Source: CAD feature listing. Evaluate the final solid. Frame: model axes, mm. A direction names the side the tool comes from. Give positions to 0.01 mm unless a question says otherwise; leave off trailing zeros. Order: outer loops, then holes, each group sorted by start corner. A loop starts at its lowest first (then second) coordinate and runs counter-clockwise, first axis right, second up.
1) Section C-C, the plane x = 3.5. Return loops of the section in (y, z) (1 decimal).
2) Material intervals for line 1 (Z direction, x = 19, y = 5.25) (1 decimal); line 2 (Y direction, x = 2, z = 7); line 3 (Z direction, x = 3, y = -2.5), sorted ascending.
3) Access query for faces 1 (the face through (19, 0, -11.112)), 2 (the face through (11, 2.413, 0)), 3 (the face through (14.713, 10, 5)). Directions: +Z, -Z, +X, -X, +Y, -Y. A direction counts if a zero-diameter tool reaches every point of the face in a straight line with its end or side. Return the directions, or none.
4) Draft query along X for faces 4 (the face through (9.22, 2.89, -8.49)), 5 (the face through (11, -8.763, -1)), 6 (the face through (7.307, 0, -12)). Return one class per face: released by +X, released by -X, zero draft, split by the parting line, or undercut.
5) First-contact query: P1, Ø11.5, axis at x = 12, z = -11, coming from the +Y side; P2, Ø1.5, axis at y = 11, z = 7.5, coming from the -X side. Flat tips, straight axial feed; report the tip coordinate or a pass-through.
6) Section A-A, the plane y = -6.5. Return loops of the section in (x, z) (1 decimal), plus the area to 3 significant figures.
7) Section B-B, the plane x = 10.25. Give the number of separate pieces and of enclosed holes in the cut face, plus the area to 4 significant figures.
8) Section D-D, the plane z = -9. Return loops of the section in (x, y) (3 decimals).
```python
from build123d import *

# Parameters (mm, degrees)
SKETCH1_W                       = 22.225
SKETCH1_H                       = 17.526
BOSS_EXTRUDE1_DEPTH             = 22.225
SKETCH2_W                       = 7.874
SKETCH2_H                       = 17.526
BOSS_EXTRUDE2_DEPTH             = 2.54
SKETCH3_W                       = 22.225
SKETCH3_H                       = 6.35
CUT_EXTRUDE1_DEPTH              = 6.35
SKETCH5_W                       = 7.874
SKETCH5_H                       = 7.9375
BOSS_EXTRUDE3_DEPTH             = 5.08
F_1_4_20_START                  = -13.6525
F_1_4_20_TAPPED_HOLE1_OUTLINE_R = 2.5527
F_1_4_20_TAPPED_HOLE1_DEPTH     = 10.4775
CUT_EXTRUDE3_REACH              = 26.382
F_1_4_20_START_2                = 4.410249561
F_1_4_20_TAPPED_HOLE2_OUTLINE_R = 2.5527
F_1_4_20_TAPPED_HOLE2_DEPTH     = 8.960808925
SKETCH21_W                      = 0.508
SKETCH21_H                      = 3.96875
BOSS_EXTRUDE4_DEPTH             = 0.02
LPATTERN1_COUNT                 = 3
LPATTERN1_PITCH                 = 6.5
SKETCH22_W                      = 0.211811424
SKETCH22_H                      = 2.54
BOSS_EXTRUDE5_DEPTH             = 0.02
LPATTERN2_COUNT                 = 5
LPATTERN2_PITCH                 = 1.016
SKETCH23_W                      = 0.254
SKETCH23_H                      = 2.54
BOSS_EXTRUDE6_DEPTH             = 0.02
LPATTERN3_COUNT                 = 5
LPATTERN3_PITCH                 = 1


# Read off the part's stored shape, not the designer's step: 1/4-20 Tapped Hole1, 1/4-20 Tapped Hole2
with BuildPart() as part:
    # Sketch1 → Boss-Extrude1 (new body)
    with BuildSketch(Plane(origin=(0, 0, 0), x_dir=(0, 0, -1), z_dir=(1, 0, 0))):
        Rectangle(SKETCH1_W, SKETCH1_H)
    extrude(amount=BOSS_EXTRUDE1_DEPTH)

    # Sketch2 → Boss-Extrude2 (add)
    with BuildSketch(Plane(origin=(0, 0, -11.1125), x_dir=(-1, 0, 0), z_dir=(0, 0, -1))):
        with Locations((-11.243689687, 0)):
            Rectangle(SKETCH2_W, SKETCH2_H)
    extrude(amount=BOSS_EXTRUDE2_DEPTH)

    # Sketch3 → Cut-Extrude1 (cut)
    with BuildSketch(Plane(origin=(0, 8.763, 0), x_dir=(1, 0, 0), z_dir=(0, 1, 0))):
        with Locations((11.1125, 0)):
            Rectangle(SKETCH3_W, SKETCH3_H)
    extrude(amount=-CUT_EXTRUDE1_DEPTH, mode=Mode.SUBTRACT)

    # Sketch5 → Boss-Extrude3 (add)
    with BuildSketch(Plane(origin=(0, 8.763, 0), x_dir=(1, 0, 0), z_dir=(0, 1, 0))):
        with Locations((10.776161326, -7.14375)):
            Rectangle(SKETCH5_W, SKETCH5_H)
    extrude(amount=BOSS_EXTRUDE3_DEPTH)

    # 1/4-20 Tapped Hole1 outline → 1/4-20 Tapped Hole1 (cut)
    with BuildSketch(Plane.XY.offset(F_1_4_20_START)):
        with Locations((11.243689687, 4.445)):
            Circle(F_1_4_20_TAPPED_HOLE1_OUTLINE_R)
    extrude(amount=F_1_4_20_TAPPED_HOLE1_DEPTH, mode=Mode.SUBTRACT)

    # Sketch6 → Cut-Extrude3 (cut, up to next)
    with BuildSketch(Plane(origin=(14.713161326, 0, 0), x_dir=(0, 0, -1), z_dir=(1, 0, 0)), mode=Mode.PRIVATE) as cut_extrude3_sk1:
        Polygon((-11.1125, 8.763), (-3.175, 13.843), (-11.1125, 13.843), align=None)
    cut_extrude3_tool1 = extrude(cut_extrude3_sk1.sketch, amount=-CUT_EXTRUDE3_REACH, mode=Mode.PRIVATE) & part.part
    add(cut_extrude3_tool1.solids().sort_by_distance((14.713161, 12.149667, 8.466667))[0], mode=Mode.SUBTRACT)

    # 1/4-20 Tapped Hole2 outline → 1/4-20 Tapped Hole2 (cut)
    with BuildSketch(Plane(origin=(0, 0, 0), x_dir=(1, 0, 0), z_dir=(0, 0.842271400661511, 0.539053696423368)).offset(F_1_4_20_START_2)):
        with Locations((10.779806469, 0.071193023)):
            Circle(F_1_4_20_TAPPED_HOLE2_OUTLINE_R)
    extrude(amount=F_1_4_20_TAPPED_HOLE2_DEPTH, mode=Mode.SUBTRACT)

    # Sketch21 → Boss-Extrude4 (add)
    with BuildSketch(Plane(origin=(0, 8.763, 0), x_dir=(1, 0, 0), z_dir=(0, 1, 0))):
        with Locations((17.4768928, 5.159375)):
            Rectangle(SKETCH21_W, SKETCH21_H)
    boss_extrude4 = extrude(amount=BOSS_EXTRUDE4_DEPTH)

    # LPattern1: Boss-Extrude4 ×3
    with Locations(*[(-i * LPATTERN1_PITCH, 0, 0) for i in range(1, LPATTERN1_COUNT)]):
        add(boss_extrude4)

    # Sketch22 → Boss-Extrude5 (add)
    with BuildSketch(Plane(origin=(0, 8.763, 0), x_dir=(1, 0, 0), z_dir=(0, 1, 0))):
        with Locations((16.354987088, 4.445)):
            Rectangle(SKETCH22_W, SKETCH22_H)
    boss_extrude5 = extrude(amount=BOSS_EXTRUDE5_DEPTH)

    # LPattern2: Boss-Extrude5 ×5
    with Locations(*[(-i * LPATTERN2_PITCH, 0, 0) for i in range(1, LPATTERN2_COUNT)]):
        add(boss_extrude5)

    # Sketch23 → Boss-Extrude6 (add)
    with BuildSketch(Plane(origin=(0, 8.763, 0), x_dir=(1, 0, 0), z_dir=(0, 1, 0))):
        with Locations((5.6198928, 4.445)):
            Rectangle(SKETCH23_W, SKETCH23_H)
    boss_extrude6 = extrude(amount=BOSS_EXTRUDE6_DEPTH)

    # LPattern3: Boss-Extrude6 ×5
    with Locations(*[(i * LPATTERN3_PITCH, 0, 0) for i in range(1, LPATTERN3_COUNT)]):
        add(boss_extrude6)


solid = part.part
```
From the geometry:
1. outline: (-8.8, -11.1) - (8.8, -11.1) - (8.8, -3.2) - (2.4, -3.2) - (2.4, 3.2) - (8.8, 3.2) - (8.8, 11.1) - (-8.8, 11.1) - close
2. line 1: z = -11.1 to -3.2, 3.2 to 11.1
2. line 2: y = -8.76 to 8.76
2. line 3: z = -11.11 to 11.11
3. face 1: -Z, +X, +Y, -Y
3. face 2: +X, -X, +Y
3. face 3: +Z, -Z, +X, +Y
4. face 4: undercut
4. face 5: zero draft
4. face 6: released by -X
5. P1: stops at y = 8.78
5. P2: stops at x = 6.84
6. outline: (0, -11.1) - (7.3, -11.1) - (7.3, -13.7) - (15.2, -13.7) - (15.2, -11.1) - (22.2, -11.1) - (22.2, 11.1) - (0, 11.1) - close
6. area: 514 mm2
7. separate pieces: 3
7. enclosed holes: 0
7. area: 329.5 mm2
8. outline: (0, -8.763) - (22.225, -8.763) - (22.225, 8.763) - (0, 8.763) - close; hole circle Ø5.105 at (11.244, 4.445)
